Geometry: final body of the model. Coordinates: model frame, mm. A direction names the side the tool comes from. Give positions to 0.01 mm unless a question says otherwise; leave off trailing zeros. Write each loop counter-clockwise with the first axis right and the second up, starting at its lowest first coordinate (ties: lowest second). Pieces come first, ordered by that corner, then holes. Notation, with made-up numbers: M 40.5,15 L 76.5,15 A4 ccw 76.5,22 Z; hole C -30,65 d4. An arc over 180 degrees is marked long. Use one line per item in the form item = value. Start each with the question number.
Item 1: Access query for faces 5 (the flat face through (-5, 56, -317.5)), 6 (the flat face through (-6, 57, -393.7)). Directions: +Z, -Z, +X, -X, +Y, -Y. A direction counts if a zero-diameter tool reaches every point of the face in a straight line with its end or side. Return the directions, or none.
Item 2: Section query D-D on y = 16.5. Return loops of the section in (x, z).
Item 3: Contact query for flat-ended pins moving along their axis: P1, Ø10, axis at y = 29, z = 214, coming from the -X side; P2, Ø2, axis at y = 94, z = -171.5, coming from the +X side; P3, Ø4, axis at x = 153.5, y = 79, coming from the -Z side. Output: stop coordinate, or through.
Item 4: Section query A-A on z = -289.5. Return loops of the section in (x, y), then the cut area to 3 significant figures.
Item 5: Material intervals for line 1 along Z through (x, y) = (-46.5, 49.5); line 2 along X through (y, z) = (70, -12); line 3 along X through (y, z) = (35.5, -178), sorted ascending. Write a range as from..to.
Item 6: Section query B-B on x = 237. Return loops of the section in (y, z), then the cut area to 3 significant figures.
Item 7: Pull-direction query (Z, two-part tool) for faces 1 (the cylindrical face through (445.74, 57.42, 382.84)), 2 (the flat face through (-5, 56, 317.5)), 3 (the flat face through (-2, 0, -318)), 4 (the cylindrical face through (-5.87, 103.44, -382.24)); classes: released by +Z, released by -Z, zero draft, split by the parting line, or undercut.
Item 8: Section query C-C on y = 92. Return loops of the section in (x, z), then the cut area to 3 significant figures.
from build123d import *

# Parameters (mm, degrees)
SKETCH1_W           = 914.4
SKETCH1_H           = 787.4
SKETCH1_W_2         = 762
SKETCH1_H_2         = 635
BOSS_EXTRUDE1_DEPTH = 114.3
FILLET2_R           = 38.1
FILLET3_R           = 38.1
FILLET4_R           = 38.1


with BuildPart() as part:
    # Sketch1 → Boss-Extrude1 (new body)
    with BuildSketch(Plane(origin=(0, 0, 0), x_dir=(1, 0, 0), z_dir=(0, 1, 0))):
        Rectangle(SKETCH1_W, SKETCH1_H)
        Rectangle(SKETCH1_W_2, SKETCH1_H_2, mode=Mode.SUBTRACT)
    extrude(amount=BOSS_EXTRUDE1_DEPTH)

    # Fillet2
    fillet2_edges = [part.edges().sort_by_distance(p)[0] for p in [
        (457.2, 57.15, 393.7),
        (-457.2, 57.15, 393.7),
        (-457.2, 57.15, -393.7),
        (457.2, 57.15, -393.7),
    ]]
    fillet(fillet2_edges, radius=FILLET2_R)

    # Fillet3
    fillet3_edges = [part.edges().sort_by_distance(p)[0] for p in [
        (457.2, 114.3, 0),
        (0, 114.3, 393.7),
        (0, 114.3, -393.7),
        (-457.2, 114.3, 0),
        (446.040768363, 114.3, -382.540768363),
        (-446.040768363, 114.3, -382.540768363),
        (-446.040768363, 114.3, 382.540768363),
        (446.040768363, 114.3, 382.540768363),
    ]]
    fillet(fillet3_edges, radius=FILLET3_R)

    # Fillet4
    fillet4_edges = [part.edges().sort_by_distance(p)[0] for p in [
        (457.2, 0, 0),
        (0, 0, 393.7),
        (-457.2, 0, 0),
        (0, 0, -393.7),
        (446.040768363, 0, -382.540768363),
        (-446.040768363, 0, -382.540768363),
        (-446.040768363, 0, 382.540768363),
        (446.040768363, 0, 382.540768363),
    ]]
    fillet(fillet4_edges, radius=FILLET4_R)


solid = part.part
Answer sheet:
q1.face_5 = +Y, -Y
q1.face_6 = -Z, +X, -X, +Y, -Y
q2.outline = M -450.49,-355.6 A31.39 ccw -419.1,-386.99 L 419.1,-386.99 A31.39 ccw 450.49,-355.6 L 450.49,355.6 A31.39 ccw 419.1,386.99 L -419.1,386.99 A31.39 ccw -450.49,355.6 Z; hole M -381,-317.5 L 381,-317.5 L 381,317.5 L -381,317.5 Z
q3.P1 = -456.98
q3.P2 = 453.3
q3.P3 = -393.69
q4.outline = M -457.2,38.1 A38.1 ccw -419.1,0 L -381,0 L -381,114.3 L -419.1,114.3 A38.1 ccw -457.2,76.2 Z; M 381,0 L 419.1,0 A38.1 ccw 457.2,38.1 L 457.2,76.2 A38.1 ccw 419.1,114.3 L 381,114.3 Z
q4.area = 16,200 mm2
q5.line_1 = -393.7..-317.5, 317.5..393.7
q5.line_2 = -457.2..-381, 381..457.2
q5.line_3 = -457.11..-381, 381..457.11
q6.outline = M 0,-355.6 A38.1 ccw 38.1,-393.7 L 76.2,-393.7 A38.1 ccw 114.3,-355.6 L 114.3,-317.5 L 0,-317.5 Z; M 0,317.5 L 114.3,317.5 L 114.3,355.6 A38.1 ccw 76.2,393.7 L 38.1,393.7 A38.1 ccw 0,355.6 Z
q6.area = 16,200 mm2
q7.face_1 = released by +Z
q7.face_2 = undercut
q7.face_3 = zero draft
q7.face_4 = released by -Z
q8.outline = M -453.77,-355.6 A34.67 ccw -419.1,-390.27 L 419.1,-390.27 A34.67 ccw 453.77,-355.6 L 453.77,355.6 A34.67 ccw 419.1,390.27 L -419.1,390.27 A34.67 ccw -453.77,355.6 Z; hole M -381,-317.5 L 381,-317.5 L 381,317.5 L -381,317.5 Z
q8.area = 223,000 mm2
